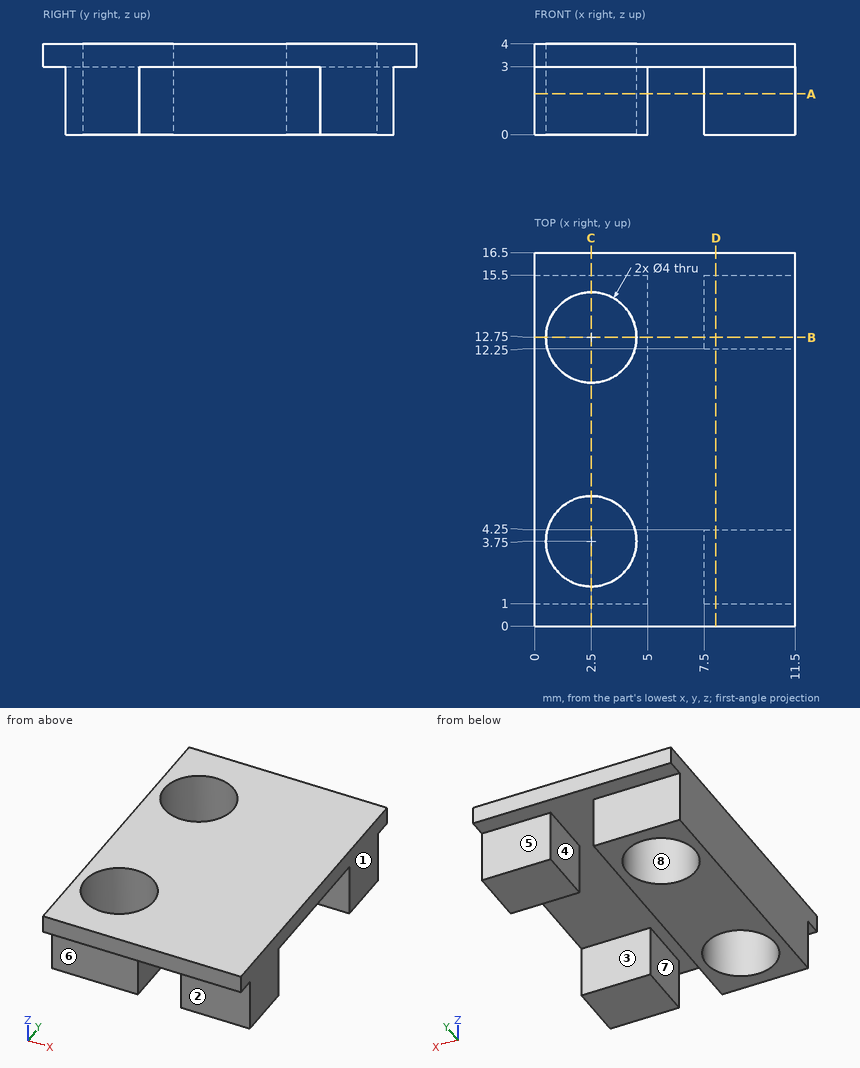
Input: dimensioned drawing with shaded views. Units: mm. Origin: part minimum x, y, z. A direction names the side the tool comes from. Round coordinates to 2 decimals unless told otherwise and drop trailing zeros. Order: outer loops, then holes, each group sorted by start corner. A loop starts at its lowest first (then second) coordinate and runs counter-clockwise, first axis right, second up. Notation, with made-up numbers: (68.25, -31) -> (94.25, -31) arc R19 cw to (94.25, 3) -> close; hole circle Ø6 at (19, 60.5). An arc over 180 degrees is marked (long way). Put each result on its own line as item: value. Start each with the question number.
Q1. Section A-A on z = 1.8. Return the cut outline in (x, y).
Q2. Section B-B on y = 12.75. Return the cut outline in (x, z), and give its area (3 significant figures).
Q3. Reachability of the marked faces 1, 2, 3, 4 and 5 from +Z, -Z, +X, -X, +Y, -Y: full face, straight path, thin tool, end or side. Return the list, or none.
Q4. First-contact query: pin 1 (4 mm diameter, centred on x = 9, y = 9.5, fed in from -Z); pin 2 (1.5 mm diameter, centred on x = 2.5, z = 2.5, fed in from +Y). Flat tips, straight axial feed; report the tip coordinate or a pass-through.
Q5. Pull-direction query (Y, two-part tool) for the marked faces 6, 7 and 8; classes: +Y half, -Y half, draft (parallel to the pull), parting line (faces both ways), or undercut.
Q6. Line query: probe 1 along Y at (x, z) = (2.5, 1); probe 2 along X at (y, z) = (3.75, 0.85); probe 3 along Y at (x, z) = (10, 1.95). Output: solid intervals per line, ascending.
Q7. Section D-D on x = 8. Return the cut outline in (y, z).
Q8. Section C-C on x = 2.5. Return the cut outline in (y, z).
Ans:
1. outline: (0, 1) -> (5, 1) -> (5, 15.5) -> (0, 15.5) -> close; (7.5, 1) -> (11.5, 1) -> (11.5, 4.25) -> (7.5, 4.25) -> close; (7.5, 12.25) -> (11.5, 12.25) -> (11.5, 15.5) -> (7.5, 15.5) -> close; hole circle Ø4 at (2.5, 3.75); hole circle Ø4 at (2.5, 12.75)
2. outline: (0, 0) -> (0.5, 0) -> (0.5, 4) -> (0, 4) -> close; (4.5, 0) -> (5, 0) -> (5, 3) -> (7.5, 3) -> (7.5, 0) -> (11.5, 0) -> (11.5, 4) -> (4.5, 4) -> close
2. area: 22.5 mm2
3. face 1: +Z, -Z, +X, +Y, -Y
3. face 2: -Z, +X, -X, -Y
3. face 3: -Z, +X
3. face 4: -Z, +Y, -Y
3. face 5: -Z, +X, -X, +Y
4. pin 1: stops at z = 3
4. pin 2: stops at y = 16.5
5. face 6: -Y half
5. face 7: draft
5. face 8: undercut
6. probe 1: y = 1 to 1.75, 5.75 to 10.75, 14.75 to 15.5
6. probe 2: x = 0 to 0.5, 4.5 to 5, 7.5 to 11.5
6. probe 3: y = 1 to 4.25, 12.25 to 15.5
7. outline: (0, 3) -> (1, 3) -> (1, 0) -> (4.25, 0) -> (4.25, 3) -> (12.25, 3) -> (12.25, 0) -> (15.5, 0) -> (15.5, 3) -> (16.5, 3) -> (16.5, 4) -> (0, 4) -> close
8. outline: (0, 3) -> (1, 3) -> (1, 0) -> (1.75, 0) -> (1.75, 4) -> (0, 4) -> close; (5.75, 0) -> (10.75, 0) -> (10.75, 4) -> (5.75, 4) -> close; (14.75, 0) -> (15.5, 0) -> (15.5, 3) -> (16.5, 3) -> (16.5, 4) -> (14.75, 4) -> close
